Autodesk Inventor part; units mm, degrees
ref_plane "YZ Plane" through (0, 0, 0) normal (1, 0, 0) x (0, 1, 0)
ref_plane "XZ Plane" through (0, 0, 0) normal (0, 1, 0) x (-1, 0, 0)
ref_plane "XY Plane" through (0, 0, 0) normal (0, 0, 1) x (1, 0, 0)
sketch "Sketch1" plane through (0, 0, 0) normal (0, 1, 0) x (-1, 0, 0)
  line L0 (0, 0) -> (-41.275, 0)
  line L1 (-41.275, 0) -> (-41.275, 41.275)
  line L2 (-41.275, 41.275) -> (0, 41.275)
  line L3 (0, 41.275) -> (0, 0)
  circle A0 centre (-20.6375, 20.6375) radius 6.35
  line L4 (0, 41.275) -> (-41.275, 0) construction
  line L5 (-41.275, 41.275) -> (0, 0) construction
  dimension "d0" = 41.275
  dimension "d1" = 41.275
  dimension "d15" = 12.7
extrude "Extrusion1" add sketch "Sketch1" along normal blind 6.35
sketch "Sketch2" plane through (0, 6.35, 0) normal (0, 1, 0) x (1, 0, 0)
  circle A0 centre (20.6375, -20.6375) radius 6.35
  circle A1 centre (20.6375, -20.6375) radius 15.875
  dimension "d4" = 12.7
  dimension "d5" = 31.75
extrude "Extrusion2" add sketch "Sketch2" along normal blind 36.5125
sketch "Sketch3" plane through (0, 6.35, 0) normal (0, 1, 0) x (1, 0, 0)
  line L0 (0, -41.275) -> (41.275, -41.275)
  line L1 (41.275, -41.275) -> (41.275, 0)
  circle A0 centre (20.6375, -20.6375) radius 15.875
  circle A1 centre (4.7625, -4.7625) radius 2.3813
  circle A2 centre (36.5125, -4.7625) radius 2.3813
  circle A3 centre (36.5125, -36.5125) radius 2.3813
  circle A4 centre (4.7625, -36.5125) radius 2.3813
  line L2 (4.7625, -36.5125) -> (4.7625, -4.7625) construction
  line L3 (4.7625, -4.7625) -> (36.5125, -4.7625) construction
  line L4 (36.5125, -4.7625) -> (36.5125, -36.5125) construction
  line L5 (36.5125, -36.5125) -> (4.7625, -36.5125) construction
  dimension "d8" = 4.7625
  dimension "d10" = 31.75
  dimension "d11" = 15.875
  dimension "d12" = 15.875
extrude "Extrusion3" cut sketch "Sketch3" against normal blind 36.5125 contours A1 | A2 | A3 | A4
properties part number "Flange Mount Linear Bearing (McMaster Part #64825K11)" material "Steel"
The model under review builds one solid part; all positions refer to its coordinate system, in mm. A direction names the side the tool comes from. Round coordinates to 2 decimals unless told otherwise and drop trailing zeros. Return JSON: item names as keys, results as strings.
1. Insertion check: P1, Ø1, axis at y = 10, z = 13.5, coming from the -X side; P2, Ø6, axis at x = 36.51, z = 4.76, coming from the +Y side; P3, Ø2, axis at x = 33.5, y = 36, coming from the +Z side. Each pin has a flat end and moves straight along its axis. Give the tip position at first contact, or say it passes through.
Answer block:
{"P1": "stops at x = 6.22", "P2": "stops at y = 6.35", "P3": "stops at z = 31.19"}
2. The part is to be moulded in two halves that separate along X. For faces 3 (the face through (2.384, 3.219, 4.658)), 4 (the face through (20, 3, 0)), 5 (the face through (17.2, 24.35, 5.14)), say which applies: +X half, -X half, draft (parallel to the pull), parting line (faces both ways), or undercut.
Answer block:
{"face 3": "undercut", "face 4": "draft", "face 5": "parting line"}
3. For faces 1 (the face through (12, 6.35, 35)), 2 (the face through (37.793, 3.219, 34.505)), list the 3-axis set-ups (+Z, -Z, +X, -X, +Y, -Y) from which the entire face can be reached by the end or side of a thin tool; tool diameter is ignored.
Answer block:
{"face 1": "+Y", "face 2": "+Y, -Y"}
4. For L1, parallel to Y at x = 31, z = 2.5; L2, parallel to Z at x = 20.5, y = 5 (3 decimals); L3, parallel to X at y = 33.5, z = 25, list the stretches that pass through material, from the lowest coordinate up. Write a range as [from, to].
Answer block:
{"L1": "y = [0, 6.35]", "L2": "z = [0, 14.289], [26.986, 41.275]", "L3": "x = [5.37, 16.02], [25.25, 35.9]"}
5. Take a section at C-C (z = 35). State how many separate pieces and enclosed holes the cut face has, then the cut area to 3 significant figures.
Answer block:
{"separate pieces": "3", "enclosed holes": "0", "area": "709 mm²"}
